Design review of the part shown in the three views and the two pictorial views. Dimensions are in mm from the part's minimum x, y and z. A direction names the side the tool comes from. Give positions to 0.01 mm unless a question says otherwise; leave off trailing zeros. Order: outer loops, then holes, each group sorted by start corner. A loop starts at its lowest first (then second) coordinate and runs counter-clockwise, first axis right, second up. Notation, with made-up numbers: M -40,76 L -27,76 A22 cw -27,100 Z; hole C 74.25,80.25 d5. An arc over 180 degrees is marked long. Answer as a JSON object with one key per item and string values.
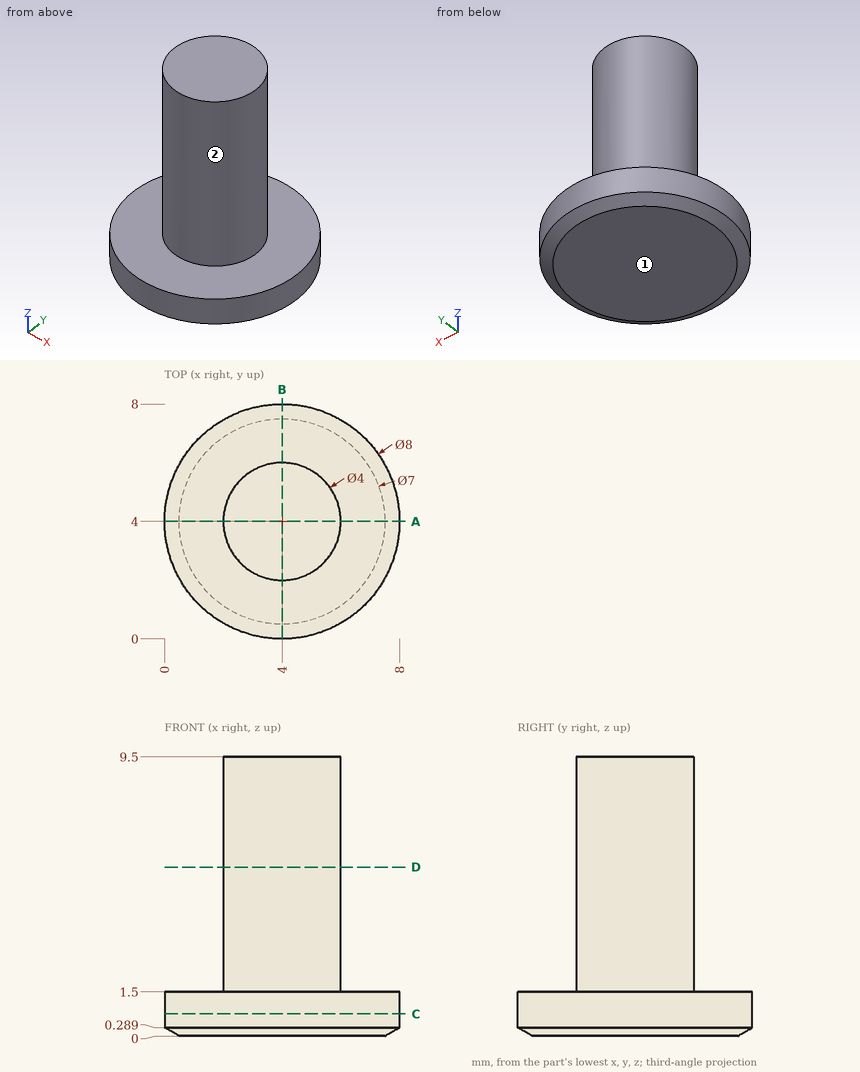
(1) Tool access review of the marked faces 1 and 2: name each direction out of +Z, -Z, +X, -X, +Y, -Y from which nothing blocks a thin tool from reaching the whole face with its end or side.
Checked values:
{"face 1": "-Z, +X, -X, +Y, -Y", "face 2": "+Z"}
(2) To check wall thickness, follow L1, parallel to Z at x = 5.5, y = 6; L2, parallel to X at y = 4.75, z = 7.25 (1 decimal); L3, parallel to Z at x = 6.5, y = 1 (1 decimal). State the ranges of each line that lie inside material, in increasing order. Write a range as from..to.
Checked values:
{"L1": "z = 0..1.5", "L2": "x = 2.1..5.9", "L3": "z = 0.2..1.5"}
(3) We need section A-A (y = 4). Write out the cut boundary in (x, z).
Checked values:
{"outline": "M 0,0.29 L 0.5,0 L 7.5,0 L 8,0.29 L 8,1.5 L 6,1.5 L 6,9.5 L 2,9.5 L 2,1.5 L 0,1.5 Z"}
(4) Insertion check: pin 1 (1.5 mm diameter, centred on x = 6, z = 1.5, fed in from -Y); pin 2 (3 mm diameter, centred on y = 4, z = 8, fed in from -X); pin 3 (1.5 mm diameter, centred on y = 4, z = 2.5, fed in from +X). Each pin has a flat end and moves straight along its axis. Give the tip position at first contact, or say it passes through.
Checked values:
{"pin 1": "stops at y = 0.2", "pin 2": "stops at x = 2", "pin 3": "stops at x = 6"}
(5) We need section D-D (z = 5.75). Write out the cut boundary in (x, y), plus the area to 3 significant figures.
Checked values:
{"outline": "C 4,4 d4", "area": "12.6 mm^2"}
(6) We need section C-C (z = 0.75). Write out the cut boundary in (x, y).
Checked values:
{"outline": "C 4,4 d8"}
